For this review, take the finished solid that the model builds, in its own axes (mm). Give positions to 0.01 mm unless a question says otherwise; leave off trailing zeros. Loops run counter-clockwise (first coordinate to the right, second up) from the corner with the lowest first, then second, coordinate; pieces in that order, holes last.
```python
from build123d import *

# Parameters (mm, degrees)
F0_R     = 38.1
F0_R_2   = 33.8298969846
F1_DEPTH = 123.825
F2_DEPTH = 9.525
F4_DEPTH = 12.7
F5_R     = 35.7824148946
F6_DEPTH = 25.4


# Not quite as in the source:
# - a fillet or chamfer that OpenCascade refuses, or shapes differently, is made with other operations: its cross-section is extruded or revolved along the edge and cut away or added


with BuildPart() as f1:
    # F0 (on Front) → F1 (new body)
    with BuildSketch(Plane.XZ):
        Circle(F0_R)
        Circle(F0_R_2, mode=Mode.SUBTRACT)
    extrude(amount=F1_DEPTH)

    # F0 (on Front) → F2 (join)
    with BuildSketch(Plane.XZ):
        Circle(F0_R)
        Circle(F0_R_2, mode=Mode.SUBTRACT)
    extrude(amount=F2_DEPTH)

    # F3: fillet of radius 6.35 on 1 edges, made by hand

    # F3_s1 → F3_t2 (revolve, cut)
    with BuildSketch(Plane.XY):
        with BuildLine():
            ThreePointArc((38.1, -117.8252892959), (36.923482669, -121.5073508209), (33.8298969846, -123.825))
            Line((33.8298969846, -123.825), (38.1, -123.825))
            Line((38.1, -123.825), (38.1, -117.8252892959))
        make_face()
    revolve(axis=Axis((0, -123.825, 0), (0, -1, 0)), mode=Mode.SUBTRACT)

    # F0 (on Front) → F4 (join)
    with BuildSketch(Plane.XZ):
        Circle(F0_R)
        Circle(F0_R_2, mode=Mode.SUBTRACT)
    extrude(amount=F4_DEPTH)

    # F5 (on Front) → F6 (join)
    with BuildSketch(Plane.XZ):
        Circle(F5_R)
    extrude(amount=F6_DEPTH)


solid = f1.part
```
Item 1: The part is to be moulded in two halves that separate along Z. For faces 1 (the flat face through (-1, 0, 1)), 2 (the flat face through (0, -25.4, 0)), 3 (the cylindrical face through (-30.235, -58.088, -23.183)), say which applies: released by +Z, released by -Z, zero draft, split by the parting line, or undercut.
Answer:
face 1: zero draft
face 2: undercut
face 3: split by the parting line
Item 2: Take a section at C-C on z = 0. Give the boundary of the cut face in (x, y) (3 decimals), and give its area (3 significant figures).
Answer:
outline: (-38.1, -117.825) arc R6.35 ccw to (-33.83, -123.825) - (-33.83, -25.4) - (33.83, -25.4) - (33.83, -123.825) arc R6.35 ccw to (38.1, -117.825) - (38.1, 0) - (-38.1, 0) - close
area: 2,760 mm2
Item 3: Take a section at B-B on x = 0. Give the boundary of the cut face in (y, z) (3 decimals).
Answer:
outline: (-123.825, -33.83) arc R6.35 ccw to (-117.825, -38.1) - (0, -38.1) - (0, 38.1) - (-117.825, 38.1) arc R6.35 ccw to (-123.825, 33.83) - (-25.4, 33.83) - (-25.4, -33.83) - close
Item 4: Take a section at D-D on y = -14.5. Give the boundary of the cut face in (x, z), and give its area (3 significant figures).
Answer:
outline: circle Ø76.2 at (0, 0)
area: 4,560 mm2
Item 5: For L1, parallel to Z at x = 0, y = -54.5; L2, parallel to Y at x = -27, z = 12.5; L3, parallel to Z at x = 18, y = -107.5, list the stretches that pass through material, from the lowest coordinate up.
Answer:
L1: z = -38.1 to -33.83, 33.83 to 38.1
L2: y = -25.4 to 0
L3: z = -33.58 to -28.64, 28.64 to 33.58
Item 6: Take a section at A-A on y = -95.5. Give the boundary of the cut face in (x, z).
Answer:
outline: circle Ø76.2 at (0, 0); hole circle Ø67.66 at (0, 0)
Item 7: Clearance check with flat-ended pins moving along their axes: pin 1 Ø3 at (x, y) = (11, -44.5) entering from +Z; pin 2 Ø10 at (y, z) = (-18.5, 27.5) entering from +X; pin 3 Ø1.5 at (y, z) = (-100.5, 13.5) entering from -X. State where each tip first meets the part, or that it passes through.
Answer:
pin 1: stops at z = 36.9
pin 2: stops at x = 30.75
pin 3: stops at x = -35.9
